Input: dimensioned drawing with shaded views. Units: mm. Origin: part minimum x, y, z. Coordinates: 2 decimals unless noted, no trailing zeros. Order: outer loops, then holes, each group sorted by start corner. A loop starts at its lowest first (then second) coordinate and runs counter-clockwise, first axis right, second up. Notation, with made-up numbers: (0.5, 0.5) - (34.5, 0.5) arc R24 cw to (34.5, 32.5) - close; hole circle Ø11 at (3, 83). An arc over 180 degrees is marked (long way). One line per question, with ' | ' between items. Start each with the question number.
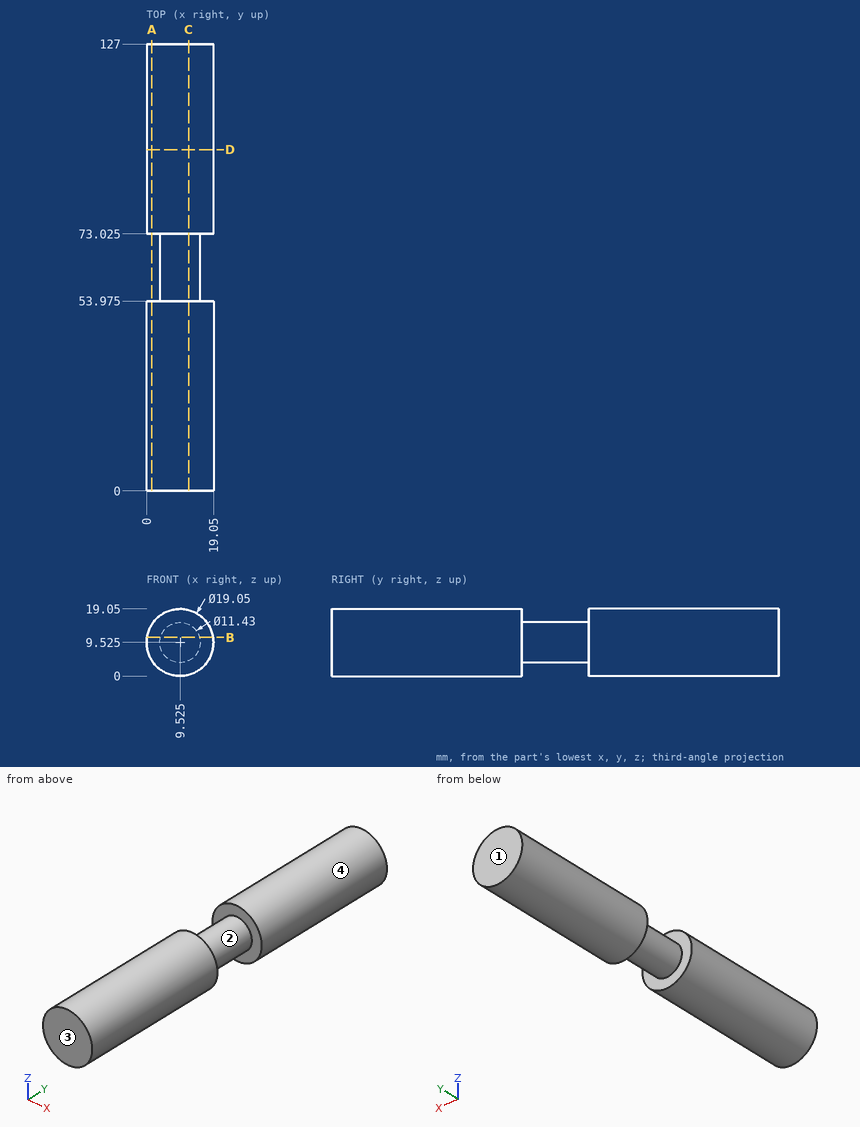
(1) Section C-C (x = 12). Output: boundary loops of the cut face in (y, z) (3 decimals), then the cut area to 3 significant figures.
(2) Material intervals for line 1 along Y through (x, z) = (8, 3) (3 decimals); line 2 along X through (y, z) = (9.5, 10), sorted ascending. Write a range as from..to.
(3) Pin query (flat end, axial travel): pin 1 (6 mm diameter, centred on y = 74.5, z = 4, fed in from +X); pin 2 (1 mm diameter, centred on y = 70, z = 12, fed in from -X). Return the tip coordinate at first contact, or that it passes through.
(4) Section A-A (x = 1.5). Output: boundary loops of the cut face in (y, z) (3 decimals), then the cut area to 3 significant figures.
(5) Section D-D (y = 97). Output: boundary loops of the cut face in (x, z) (3 decimals).
(6) Draft query along Y for the marked faces 1, 2, 3 and 4. Return one class per face: +Y half, -Y half, draft (parallel to the pull), parting line (faces both ways), or undercut.
(7) Section B-B (z = 11). Output: boundary loops of the cut face in (x, y) (3 decimals), then the cut area to 3 significant figures.
Worked answers:
1) outline: (0, 0.327) - (53.975, 0.327) - (53.975, 4.374) - (73.025, 4.374) - (73.025, 0.327) - (127, 0.327) - (127, 18.723) - (73.025, 18.723) - (73.025, 14.676) - (53.975, 14.676) - (53.975, 18.723) - (0, 18.723) - close | area: 2,180 mm²
2) line 1: y = 0..53.975, 73.025..127 | line 2: x = 0.01..19.04
3) pin 1: stops at x = 18.71 | pin 2: stops at x = 4.16
4) outline: (0, 4.394) - (53.975, 4.394) - (53.975, 14.656) - (0, 14.656) - close; (73.025, 4.394) - (127, 4.394) - (127, 14.656) - (73.025, 14.656) - close | area: 1,110 mm²
5) outline: circle Ø19.05 at (9.525, 9.525)
6) face 1: +Y half | face 2: undercut | face 3: -Y half | face 4: draft
7) outline: (0.115, 0) - (18.935, 0) - (18.935, 53.975) - (15.046, 53.975) - (15.046, 73.025) - (18.935, 73.025) - (18.935, 127) - (0.115, 127) - (0.115, 73.025) - (4.004, 73.025) - (4.004, 53.975) - (0.115, 53.975) - close | area: 2,240 mm²
